```python
from build123d import *

# Parameters (mm, degrees)
SKETCH2_W           = 88.33
SKETCH2_H           = 80
BOSS_EXTRUDE1_DEPTH = 6.35
SKETCH3_W           = 6.45
SKETCH3_H           = 13.333333334
CUT_EXTRUDE1_DEPTH  = 60.923866072
M5_TAPPED_HOLE1_D   = 4.2
CUT_EXTRUDE2_DEPTH  = 10
CUT_EXTRUDE3_REACH  = 61.924


with BuildPart() as part:
    # Sketch2 → Boss-Extrude1 (new body)
    with BuildSketch(Plane(origin=(0, 0, 0), x_dir=(1, 0, 0), z_dir=(0, 1, 0))):
        Rectangle(SKETCH2_W, SKETCH2_H)
    extrude(amount=BOSS_EXTRUDE1_DEPTH)

    # Sketch3 → Cut-Extrude1 (cut, through all)
    with BuildSketch(Plane(origin=(0, 6.35, 0), x_dir=(1, 0, 0), z_dir=(0, 1, 0))):
        with Locations((40.94, -20)):
            Rectangle(SKETCH3_W, SKETCH3_H)
        with Locations((40.94, 20)):
            Rectangle(SKETCH3_W, SKETCH3_H)
    extrude(amount=-CUT_EXTRUDE1_DEPTH, mode=Mode.SUBTRACT)

    # M5 Tapped Hole1 (through all)
    with Locations(Plane(origin=(0, 6.35, 0), x_dir=(1, 0, 0), z_dir=(0, 1, 0))):
        with Locations((-36.165, 32), (27.835, 32), (-36.165, -32), (27.835, -32)):
            Hole(M5_TAPPED_HOLE1_D / 2)

    # Sketch7 → Cut-Extrude2 (cut)
    with BuildSketch(Plane(origin=(0, 6.35, 0), x_dir=(1, 0, 0), z_dir=(0, 1, 0))):
        with BuildLine():
            Line((-26.165, 32), (-14.165, 32))
            ThreePointArc((-14.165, 32), (-10.629466094, 30.535533906), (-9.165, 27))
            Line((-9.165, 27), (-9.165, 10))
            ThreePointArc((-9.165, 10), (-10.629466094, 6.464466094), (-14.165, 5))
            Line((-14.165, 5), (-31.165, 5))
            ThreePointArc((-31.165, 5), (-34.700533906, 6.464466094), (-36.165, 10))
            Line((-36.165, 10), (-36.165, 22))
            ThreePointArc((-36.165, 22), (-29.093932188, 24.928932188), (-26.165, 32))
        make_face()
        with BuildLine():
            Line((-31.165, -5), (-14.165, -5))
            ThreePointArc((-14.165, -5), (-10.629466094, -6.464466094), (-9.165, -10))
            Line((-9.165, -10), (-9.165, -27))
            ThreePointArc((-9.165, -27), (-10.629466094, -30.535533906), (-14.165, -32))
            Line((-14.165, -32), (-26.165, -32))
            ThreePointArc((-26.165, -32), (-29.093932188, -24.928932188), (-36.165, -22))
            Line((-36.165, -22), (-36.165, -10))
            ThreePointArc((-36.165, -10), (-34.700533906, -6.464466094), (-31.165, -5))
        make_face()
        with BuildLine():
            Line((27.835, 22), (27.835, 10))
            ThreePointArc((27.835, 10), (26.370533906, 6.464466094), (22.835, 5))
            Line((22.835, 5), (5.835, 5))
            ThreePointArc((5.835, 5), (2.299466094, 6.464466094), (0.835, 10))
            Line((0.835, 10), (0.835, 27))
            ThreePointArc((0.835, 27), (2.299466094, 30.535533906), (5.835, 32))
            Line((5.835, 32), (17.835, 32))
            ThreePointArc((17.835, 32), (20.763932188, 24.928932188), (27.835, 22))
        make_face()
        with BuildLine():
            Line((17.835, -32), (5.835, -32))
            ThreePointArc((5.835, -32), (2.299466094, -30.535533906), (0.835, -27))
            Line((0.835, -27), (0.835, -10))
            ThreePointArc((0.835, -10), (2.299466094, -6.464466094), (5.835, -5))
            Line((5.835, -5), (22.835, -5))
            ThreePointArc((22.835, -5), (26.370533906, -6.464466094), (27.835, -10))
            Line((27.835, -10), (27.835, -22))
            ThreePointArc((27.835, -22), (20.763932188, -24.928932188), (17.835, -32))
        make_face()
    extrude(amount=-CUT_EXTRUDE2_DEPTH, mode=Mode.SUBTRACT)

    # Sketch8 → Cut-Extrude3 (cut, up to next)
    with BuildSketch(Plane(origin=(0, 6.35, 0), x_dir=(1, 0, 0), z_dir=(0, 1, 0)), mode=Mode.PRIVATE) as cut_extrude3_sk1:
        with BuildLine():
            Line((17.835, 45), (17.835, 32))
            ThreePointArc((17.835, 32), (20.763932188, 24.928932188), (27.835, 22))
            Line((27.835, 22), (27.835, -22))
            ThreePointArc((27.835, -22), (20.763932188, -24.928932188), (17.835, -32))
            Line((17.835, -32), (17.835, -45))
            Line((17.835, -45), (-49.165, -45))
            Line((-49.165, -45), (-49.165, 45))
            Line((-49.165, 45), (17.835, 45))
        make_face()
    cut_extrude3_tool1 = extrude(cut_extrude3_sk1.sketch, amount=-CUT_EXTRUDE3_REACH, mode=Mode.PRIVATE) & part.part
    add(cut_extrude3_tool1.solids().sort_by_distance((-12.82853, 6.35, 0))[0], mode=Mode.SUBTRACT)


solid = part.part
```
Check sheet for the modelled part. Datum: model origin and axes. Units: mm. A direction names the side the tool comes from. Coordinates: 2 decimals unless noted, no trailing zeros. Loops run counter-clockwise (first coordinate to the right, second up) from the corner with the lowest first, then second, coordinate; pieces in that order, holes last. Notation, with made-up numbers: M 78,36 L 126,36 A13 ccw 126,40 Z; hole C 53.25,55.5 d9. An arc over 180 degrees is marked long. Answer as a JSON object with one key per item and string values.
1. Sectioned sample at D-D on z = 3. Record the cut outline in (x, y) (3 decimals).
Outcome:
{"outline": "M 27.835,0 L 44.165,0 L 44.165,6.35 L 27.835,6.35 Z"}
2. Scan lines: L1, parallel to Z at x = 41, y = 3.5; L2, parallel to Z at x = 27.5, y = 1.75; L3, parallel to X at y = 1.25, z = 32 (3 decimals). Record each from-to range of solid material in increasing order. Write a range as from..to.
Outcome:
{"L1": "-40..-26.67, -13.33..13.33, 26.67..40", "L2": "-40..-34.07, -29.93..-22.01, 22.01..29.93, 34.07..40", "L3": "17.835..25.735, 29.935..44.165"}
3. Sectioned sample at C-C on z = -16.5. Record the cut outline in (x, y) (3 decimals), and give its area (3 significant figures).
Outcome:
{"outline": "M 27.835,0 L 37.715,0 L 37.715,6.35 L 27.835,6.35 Z", "area": "62.7 mm²"}
4. Sectioned sample at B-B on y = 5. Record the cut outline in (x, z) (3 decimals).
Outcome:
{"outline": "M 17.835,-40 L 44.165,-40 L 44.165,-26.667 L 37.715,-26.667 L 37.715,-13.333 L 44.165,-13.333 L 44.165,13.333 L 37.715,13.333 L 37.715,26.667 L 44.165,26.667 L 44.165,40 L 17.835,40 L 17.835,32 A10 ccw 27.835,22 L 27.835,-22 A10 ccw 17.835,-32 Z; hole C 27.835,-32 d4.2; hole C 27.835,32 d4.2"}
5. Access from +Z, -Z, +X, -X, +Y, -Y to the whole of each face (thin tool, end or side, straight path). Record for faces 5 (the flat face through (31, 0, -1)), 6 (the cylindrical face through (20.842, 3.219, 24.852)), 7 (the flat face through (41, 3, -13.333)).
Outcome:
{"face 5": "+Z, -Z, +X, -X, -Y", "face 6": "-X, +Y, -Y", "face 7": "+X, +Y, -Y"}
6. Sectioned sample at A-A on x = 38.75. Record the cut outline in (y, z), and give its area (3 significant figures).
Outcome:
{"outline": "M 0,-40 L 6.35,-40 L 6.35,-26.67 L 0,-26.67 Z; M 0,-13.33 L 6.35,-13.33 L 6.35,13.33 L 0,13.33 Z; M 0,26.67 L 6.35,26.67 L 6.35,40 L 0,40 Z", "area": "339 mm²"}
7. Depth check by flat-ended pin: P1, Ø3, axis at y = 2, z = 20, coming from the +X side (3 decimals); P2, Ø3, axis at y = 4, z = 6, coming from the -X side (3 decimals); P3, Ø4, axis at x = 27.835, z = 32, coming from the -Y side. Enter the tip coordinate at first touch or a pass-through.
Outcome:
{"P1": "x = 37.715", "P2": "x = 27.835", "P3": "through"}
8. Release check for a two-part mould opening along X. For faces 1 (the flat face through (31, 3, -40)), 2 (the cylindrical face through (26.866, 3.131, -30.137)), 3 (the flat face through (37.715, 3, 20)), 4 (the cylindrical face through (20.687, 3.219, -25.007)) record: pulls with the +X half, pulls with the -X half, needs draft (parallel to the pull), parting line crosses it, or undercut.
Outcome:
{"face 1": "needs draft", "face 2": "undercut", "face 3": "pulls with the +X half", "face 4": "pulls with the -X half"}
